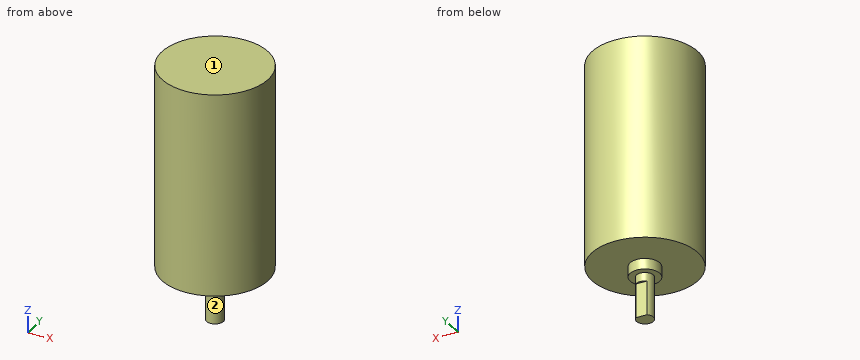
```python
from build123d import *

# Parameters (mm, degrees)
F0_R     = 12.5
F1_DEPTH = 47.8
F2_R     = 3.5
F3_DEPTH = 2.5
F4_R     = 2
F5_DEPTH = 12.5
F7_DEPTH = 8


with BuildPart() as f1:
    # F0 (on Top) → F1 (new body)
    with BuildSketch(Plane.XY):
        Circle(F0_R)
    extrude(amount=F1_DEPTH)

    # F2 (on face) → F3 (join)
    with BuildSketch(Plane(origin=(0, 0, 0), x_dir=(1, 0, 0), z_dir=(0, 0, -1))):
        Circle(F2_R)
    extrude(amount=F3_DEPTH)

    # F4 (on face) → F5 (join)
    with BuildSketch(Plane(origin=(0, 0, 0), x_dir=(1, 0, 0), z_dir=(0, 0, -1))):
        Circle(F4_R)
    extrude(amount=F5_DEPTH)

    # F6 (on face) → F7 (cut)
    with BuildSketch(Plane(origin=(0, 0, -12.5), x_dir=(1, 0, 0), z_dir=(0, 0, -1))):
        with BuildLine():
            ThreePointArc((-1.322876, -1.5), (0, -2), (1.322876, -1.5))
            Line((1.322876, -1.5), (-1.322876, -1.5))
        make_face()
    extrude(amount=-F7_DEPTH, mode=Mode.SUBTRACT)


solid = f1.part
```
Geometry check sheet. Reference: the model listing, model coordinates, mm. Face numbers are marked on the shaded views. A direction names the side the tool comes from. Give positions to 0.01 mm unless a question says otherwise; leave off trailing zeros. Write each loop counter-clockwise with the first axis right and the second up, starting at its lowest first coordinate (ties: lowest second). Pieces come first, ordered by that corner, then holes. Notation, with made-up numbers: (10.5, 31) -> (14.5, 31) arc R14 ccw to (14.5, 54) -> close; hole circle Ø11 at (59, -24). An arc over 180 degrees is marked (long way). One line per question, with ' | ' between items.
Item 1: Access from +Z, -Z, +X, -X, +Y, -Y to the whole of each face (thin tool, end or side, straight path). Record for the marked faces 1 and 2.
Determined:
face 1: +Z, +X, -X, +Y, -Y | face 2: -Z
Item 2: Sectioned sample at D-D, the plane y = -9.5. Record the boundary of the cut face in (x, z).
Determined:
outline: (-8.12, 0) -> (8.12, 0) -> (8.12, 47.8) -> (-8.12, 47.8) -> close
Item 3: Sectioned sample at C-C, the plane z = 8. Record the boundary of the cut face in (x, y), plus the area to 3 significant figures.
Determined:
outline: circle Ø25 at (0, 0) | area: 491 mm^2
Item 4: Depth check by flat-ended pin: pin 1 (10 mm diameter, centred on y = -9.5, z = 18.5, fed in from +X); pin 2 (4 mm diameter, centred on y = -1, z = 16.5, fed in from +X); pin 3 (1.5 mm diameter, centred on y = -1.5, z = 8.5, fed in from -X); pin 4 (3 mm diameter, centred on x = 0, z = -7.5, fed in from +Y). Enter the tip coordinate at first touch or a pass-through.
Determined:
pin 1: x = 11.66 | pin 2: x = 12.5 | pin 3: x = -12.48 | pin 4: y = 1.5
Item 5: Scan lines: line 1 along Y through (x, z) = (0.5, 34.5); line 2 along Z through (x, y) = (0, 9.5); line 3 along X through (y, z) = (-4, 19). Record each from-to range of solid material in increasing order.
Determined:
line 1: -12.49 to 12.49 | line 2: 0 to 47.8 | line 3: -11.84 to 11.84
Item 6: Sectioned sample at B-B, the plane x = 0. Record the boundary of the cut face in (y, z).
Determined:
outline: (-12.5, 0) -> (-3.5, 0) -> (-3.5, -2.5) -> (-2, -2.5) -> (-2, -12.5) -> (1.5, -12.5) -> (1.5, -4.5) -> (2, -4.5) -> (2, -2.5) -> (3.5, -2.5) -> (3.5, 0) -> (12.5, 0) -> (12.5, 47.8) -> (-12.5, 47.8) -> close
Item 7: Sectioned sample at A-A, the plane y = 0. Record the boundary of the cut face in (x, z), plus the area to 3 significant figures.
Determined:
outline: (-12.5, 0) -> (-3.5, 0) -> (-3.5, -2.5) -> (-2, -2.5) -> (-2, -12.5) -> (2, -12.5) -> (2, -2.5) -> (3.5, -2.5) -> (3.5, 0) -> (12.5, 0) -> (12.5, 47.8) -> (-12.5, 47.8) -> close | area: 1,250 mm^2
